from build123d import *

# Parameters (mm, degrees)
F1_DEPTH      = 609.6
F1_DEPTH_BACK = 152.4
F2_DEPTH      = 457.2
F3_DEPTH      = 457.2
F5_DEPTH      = 2540


with BuildPart() as f1:
    # F0 (on Front) → F1 (new body, two sides)
    with BuildSketch(Plane.XZ) as f1_sk:
        Polygon((148.710757494, 22.0376051942), (-1121.289242506, 22.0376051942), (-1121.289242506, 6.7976051942), (-1060.329242506, 6.7976051942), (-979.049242506, 6.7976051942), (-940.949242506, 6.7976051942), (-928.249242506, 6.7976051942), (-623.449242506, 6.7976051942), (-610.749242506, 6.7976051942), (-361.829242506, 6.7976051942), (-349.129242506, 6.7976051942), (-44.329242506, 6.7976051942), (-31.629242506, 6.7976051942), (6.470757494, 6.7976051942), (87.750757494, 6.7976051942), (148.710757494, 6.7976051942), align=None)
    extrude(amount=-F1_DEPTH)
    extrude(f1_sk.sketch, amount=F1_DEPTH_BACK)

    # F0 (on Front) → F2 (join)
    with BuildSketch(Plane.XZ):
        Polygon((-979.049242506, 6.7976051942), (-1060.329242506, 6.7976051942), (-1060.329242506, -69.4023948058), (-1045.089242506, -69.4023948058), (-1045.089242506, -348.8023948058), (-994.289242506, -348.8023948058), (-994.289242506, -298.0023948058), (-994.289242506, -282.7623948058), (-994.289242506, -82.1023948058), (-994.289242506, -69.4023948058), (-979.049242506, -69.4023948058), align=None)
        Polygon((87.750757494, -69.4023948058), (87.750757494, 6.7976051942), (6.470757494, 6.7976051942), (6.470757494, -69.4023948058), (21.710757494, -69.4023948058), (21.710757494, -82.1023948058), (21.710757494, -282.7623948058), (21.710757494, -298.0023948058), (21.710757494, -348.8023948058), (72.510757494, -348.8023948058), (72.510757494, -69.4023948058), align=None)
    extrude(amount=-F2_DEPTH)

    # F0 (on Front) → F3 (join)
    with BuildSketch(Plane.XZ):
        Polygon((-486.289242506, -282.7623948058), (-994.289242506, -282.7623948058), (-994.289242506, -298.0023948058), (-486.289242506, -298.0023948058), (21.710757494, -298.0023948058), (21.710757494, -282.7623948058), align=None)
    extrude(amount=-F3_DEPTH)

    # F4 (on face) → F5 (cut)
    with BuildSketch(Plane(origin=(-1060.329242506, 0, 0), x_dir=(0, -1, 0), z_dir=(-1, 0, 0))):
        Polygon((-457.2, -270.0623948058), (-409.3666133917, -270.0623948058), (-359.05659291, -187.2455320743), (-457.2, -69.4023948058), align=None)
        Polygon((-374.5619450508, -69.4023948058), (-324.2021632287, -129.8705898486), (-287.4686281641, -69.4023948058), align=None)
        Polygon((-228.6, -94.8023948058), (-281.2405547119, -181.4556211801), (-228.6, -244.6623948058), (-175.9594452881, -181.4556211801), align=None)
        Polygon((-82.6380549492, -69.4023948058), (-169.7313718359, -69.4023948058), (-132.9978367713, -129.8705898486), align=None)
        Polygon((-98.14340709, -187.2455320743), (-47.8333866083, -270.0623948058), (0, -270.0623948058), (0, -69.4023948058), align=None)
        Polygon((-167.1158501306, -270.0623948058), (-122.1321394847, -270.0623948058), (-141.1050156067, -238.8305634058), align=None)
        Polygon((-316.0949843933, -238.8305634058), (-335.0678605153, -270.0623948058), (-290.0841498694, -270.0623948058), align=None)
        Polygon((-359.756060055, -310.7023948058), (-382.9012471236, -348.8023948058), (-74.2987528764, -348.8023948058), (-97.443939945, -310.7023948058), align=None)
        Polygon((-457.2, -310.7023948058), (-457.2, -348.8023948058), (-434.0548129315, -310.7023948058), align=None)
        Polygon((-23.1451870685, -310.7023948058), (0, -348.8023948058), (0, -310.7023948058), align=None)
        Polygon((-47.8333866083, -270.0623948058), (-23.1451870685, -310.7023948058), (0, -310.7023948058), (0, -270.0623948058), align=None)
        Polygon((-457.2, -310.7023948058), (-434.0548129315, -310.7023948058), (-409.3666133917, -270.0623948058), (-457.2, -270.0623948058), align=None)
    extrude(amount=-F5_DEPTH, mode=Mode.SUBTRACT)


solid = f1.part
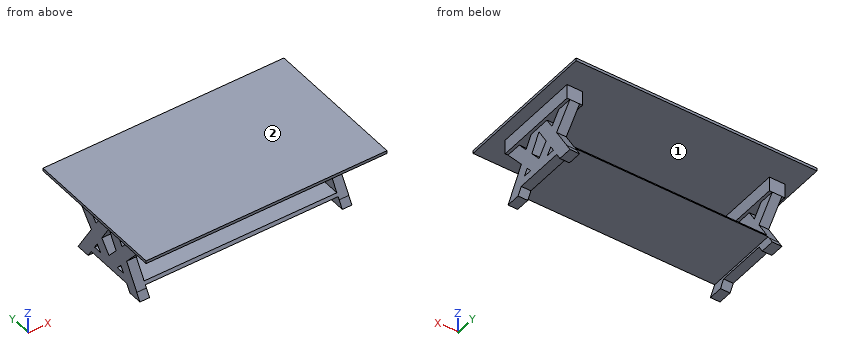
The listing builds one solid part. Answer for the finished solid, in the listing's coordinates (mm). Face numbers are marked on the shaded views. Coordinates: 2 decimals unless noted, no trailing zeros. Order: outer loops, then holes, each group sorted by start corner. A loop starts at its lowest first (then second) coordinate and runs counter-clockwise, first axis right, second up. Notation, with made-up numbers: (85.5, 78.5) -> (115.5, 78.5) arc R25 ccw to (115.5, 107.5) -> close; hole circle Ø9 at (-25.75, -27.75). An arc over 180 degrees is marked (long way). Answer in a Markdown table with one row per item. Add a question column.
Item 1: Find section B-B (z = -29). Write down the section's boundary in (x, y).
Item 2: Find the intervals of material crossed by L1, parallel to X at y = 95, z = -262.5; L2, parallel to Z at x = -440, y = 363.5; L3, parallel to X at y = 454, z = -2, in increasing order. Write a range as from..to.
Item 3: Find section C-C (x = 59). State how many separate pieces and enclosed holes the cut face has, then the cut area to 3 significant figures.
Item 4: Determine the mould class of the marked faces 1 and 2 for opening direction X: +X half, -X half, draft (parallel to the pull), parting line (faces both ways), or undercut.
Item 5: Each of these flat-tipped pins is pushed along its axis until it touches: P1, Ø23, axis at x = 57, z = -36, coming from the +Y side; P2, Ø1, axis at x = -983.5, y = 362, coming from the -Z side; P3, Ø1.5, axis at x = -874.5, y = -1.5, coming from the -Z side. Where does it stop, or does it pass through?
Item 6: Find section A-A (x = -785). Write down the section's boundary in (y, z).
Result set:
| question | item | result |
|---|---|---|
| 1 | outline | (-1060.33, 0) -> (-979.05, 0) -> (-979.05, 457.2) -> (-1060.33, 457.2) -> close; (6.47, 0) -> (87.75, 0) -> (87.75, 457.2) -> (6.47, 457.2) -> close |
| 2 | L1 | x = -1045.09..-994.29, 21.71..72.51 |
| 2 | L2 | z = -298..-282.76, 6.8..22.04 |
| 2 | L3 | x = -1060.33..-979.05, 6.47..87.75 |
| 3 | separate pieces | 1 |
| 3 | enclosed holes | 5 |
| 3 | area | 121,000 mm² |
| 4 | face 1 | undercut |
| 4 | face 2 | draft |
| 5 | P1 | stops at y = 457.2 |
| 5 | P2 | stops at z = -298 |
| 5 | P3 | stops at z = 6.8 |
| 6 | outline | (-152.4, 6.8) -> (609.6, 6.8) -> (609.6, 22.04) -> (-152.4, 22.04) -> close; (30.86, -298) -> (426.34, -298) -> (417.08, -282.76) -> (40.12, -282.76) -> close |
